```python
from build123d import *

# Parameters (mm, degrees)
F1_DEPTH = 20
F2_R     = 1.5
F3_DEPTH = 5.2010001


with BuildPart() as f1:
    # F0 (on Top) → F1 (new body)
    with BuildSketch(Plane.XY):
        with BuildLine():
            Line((-17.7, 10.1), (-17.7, 0))
            Line((-17.7, 0), (-17.7, -6.1))
            ThreePointArc((-17.7, -6.1), (-17.4363961031, -6.7363961031), (-16.8, -7))
            ThreePointArc((-16.8, -7), (-16.1636038969, -6.7363961031), (-15.9, -6.1))
            Line((-15.9, -6.1), (-15.9, -2.9281131564))
            Line((-15.9, -2.9281131564), (-15.9, -0.2))
            ThreePointArc((-15.9, -0.2), (-15.8414213562, -0.0585786438), (-15.7, 0))
            Line((-15.7, 0), (-13.1, 0))
            ThreePointArc((-13.1, 0), (-12.9585786438, -0.0585786438), (-12.9, -0.2))
            Line((-12.9, -0.2), (-12.9, -2.9281131564))
            Line((-12.9, -2.9281131564), (-12.9, -6.1))
            ThreePointArc((-12.9, -6.1), (-12.6363961031, -6.7363961031), (-12, -7))
            ThreePointArc((-12, -7), (-11.3636038969, -6.7363961031), (-11.1, -6.1))
            Line((-11.1, -6.1), (-11.1, -2.9281131564))
            ThreePointArc((-11.1, -2.9281131564), (-11.0414213562, -2.7866918002), (-10.9, -2.7281131564))
            Line((-10.9, -2.7281131564), (-10.7902640884, -2.7281131564))
            ThreePointArc((-10.7902640884, -2.7281131564), (-10.6130008648, -2.6207292974), (-10.6260897314, -2.4138906521))
            ThreePointArc((-10.6260897314, -2.4138906521), (-9.6, -0.45), (-8.5739102686, -2.4138906521))
            ThreePointArc((-8.5739102686, -2.4138906521), (-8.5869991352, -2.6207292974), (-8.4097359116, -2.7281131564))
            Line((-8.4097359116, -2.7281131564), (-8.3, -2.7281131564))
            ThreePointArc((-8.3, -2.7281131564), (-8.1585786438, -2.7866918002), (-8.1, -2.9281131564))
            Line((-8.1, -2.9281131564), (-8.1, -6.1))
            ThreePointArc((-8.1, -6.1), (-7.8363961031, -6.7363961031), (-7.2, -7))
            ThreePointArc((-7.2, -7), (-6.5636038969, -6.7363961031), (-6.3, -6.1))
            Line((-6.3, -6.1), (-6.3, -0.2))
            ThreePointArc((-6.3, -0.2), (-6.2414213562, -0.0585786438), (-6.1, 0))
            Line((-6.1, 0), (6.1, 0))
            ThreePointArc((6.1, 0), (6.2414213562, -0.0585786438), (6.3, -0.2))
            Line((6.3, -0.2), (6.3, -6.1))
            ThreePointArc((6.3, -6.1), (6.5636038969, -6.7363961031), (7.2, -7))
            ThreePointArc((7.2, -7), (7.8363961031, -6.7363961031), (8.1, -6.1))
            Line((8.1, -6.1), (8.1, -2.9281131564))
            ThreePointArc((8.1, -2.9281131564), (8.1585786438, -2.7866918002), (8.3, -2.7281131564))
            Line((8.3, -2.7281131564), (8.4097359116, -2.7281131564))
            ThreePointArc((8.4097359116, -2.7281131564), (8.5869991352, -2.6207292974), (8.5739102686, -2.4138906521))
            ThreePointArc((8.5739102686, -2.4138906521), (9.6, -0.45), (10.6260897314, -2.4138906521))
            ThreePointArc((10.6260897314, -2.4138906521), (10.6130008648, -2.6207292974), (10.7902640884, -2.7281131564))
            Line((10.7902640884, -2.7281131564), (10.9, -2.7281131564))
            ThreePointArc((10.9, -2.7281131564), (11.0414213562, -2.7866918002), (11.1, -2.9281131564))
            Line((11.1, -2.9281131564), (11.1, -6.1))
            ThreePointArc((11.1, -6.1), (11.3636038969, -6.7363961031), (12, -7))
            ThreePointArc((12, -7), (12.6363961031, -6.7363961031), (12.9, -6.1))
            Line((12.9, -6.1), (12.9, -2.9281131564))
            Line((12.9, -2.9281131564), (12.9, -0.2))
            ThreePointArc((12.9, -0.2), (12.9585786438, -0.0585786438), (13.1, 0))
            Line((13.1, 0), (15.7, 0))
            ThreePointArc((15.7, 0), (15.8414213562, -0.0585786438), (15.9, -0.2))
            Line((15.9, -0.2), (15.9, -2.9281131564))
            Line((15.9, -2.9281131564), (15.9, -6.1))
            ThreePointArc((15.9, -6.1), (16.1636038969, -6.7363961031), (16.8, -7))
            ThreePointArc((16.8, -7), (17.4363961031, -6.7363961031), (17.7, -6.1))
            Line((17.7, -6.1), (17.7, 0))
            Line((17.7, 0), (17.7, 10.1))
            ThreePointArc((17.7, 10.1), (17.4363961031, 10.7363961031), (16.8, 11))
            ThreePointArc((16.8, 11), (16.1636038969, 10.7363961031), (15.9, 10.1))
            Line((15.9, 10.1), (15.9, 2.2532098395))
            ThreePointArc((15.9, 2.2532098395), (15.8239660819, 2.096262681), (15.6536758945, 2.0586485965))
            Line((15.6536758945, 2.0586485965), (13.0536758945, 2.6776962156))
            ThreePointArc((13.0536758945, 2.6776962156), (12.9430528415, 2.7482913767), (12.9, 2.8722574585))
            Line((12.9, 2.8722574585), (12.9, 10.1))
            ThreePointArc((12.9, 10.1), (12.6363961031, 10.7363961031), (12, 11))
            ThreePointArc((12, 11), (11.3636038969, 10.7363961031), (11.1, 10.1))
            Line((11.1, 10.1), (11.1, 3.3960669823))
            ThreePointArc((11.1, 3.3960669823), (11.0239660819, 3.2391198239), (10.8536758945, 3.2015057394))
            Line((10.8536758945, 3.2015057394), (8.2536758945, 3.8205533584))
            ThreePointArc((8.2536758945, 3.8205533584), (8.1430528415, 3.8911485195), (8.1, 4.0151146014))
            Line((8.1, 4.0151146014), (8.1, 10.1))
            ThreePointArc((8.1, 10.1), (7.8363961031, 10.7363961031), (7.2, 11))
            ThreePointArc((7.2, 11), (6.5636038969, 10.7363961031), (6.3, 10.1))
            Line((6.3, 10.1), (6.3, 4.5389241252))
            ThreePointArc((6.3, 4.5389241252), (6.2239660819, 4.3819769667), (6.0536758945, 4.3443628823))
            Line((6.0536758945, 4.3443628823), (3.4536758945, 4.9634105013))
            ThreePointArc((3.4536758945, 4.9634105013), (3.3430528415, 5.0340056624), (3.3, 5.1579717442))
            Line((3.3, 5.1579717442), (3.3, 10.1))
            ThreePointArc((3.3, 10.1), (3.0363961031, 10.7363961031), (2.4, 11))
            ThreePointArc((2.4, 11), (1.7636038969, 10.7363961031), (1.5, 10.1))
            Line((1.5, 10.1), (1.5, 5.2))
            ThreePointArc((1.5, 5.2), (1.4414213562, 5.0585786438), (1.3, 5))
            Line((1.3, 5), (-1.3, 5))
            ThreePointArc((-1.3, 5), (-1.4414213562, 5.0585786438), (-1.5, 5.2))
            Line((-1.5, 5.2), (-1.5, 10.1))
            ThreePointArc((-1.5, 10.1), (-1.7636038969, 10.7363961031), (-2.4, 11))
            ThreePointArc((-2.4, 11), (-3.0363961031, 10.7363961031), (-3.3, 10.1))
            Line((-3.3, 10.1), (-3.3, 5.1579717442))
            ThreePointArc((-3.3, 5.1579717442), (-3.3430528415, 5.0340056624), (-3.4536758945, 4.9634105013))
            Line((-3.4536758945, 4.9634105013), (-6.0536758945, 4.3443628823))
            ThreePointArc((-6.0536758945, 4.3443628823), (-6.2239660819, 4.3819769667), (-6.3, 4.5389241252))
            Line((-6.3, 4.5389241252), (-6.3, 10.1))
            ThreePointArc((-6.3, 10.1), (-6.5636038969, 10.7363961031), (-7.2, 11))
            ThreePointArc((-7.2, 11), (-7.8363961031, 10.7363961031), (-8.1, 10.1))
            Line((-8.1, 10.1), (-8.1, 4.0151146014))
            ThreePointArc((-8.1, 4.0151146014), (-8.1430528415, 3.8911485195), (-8.2536758945, 3.8205533584))
            Line((-8.2536758945, 3.8205533584), (-10.8536758945, 3.2015057394))
            ThreePointArc((-10.8536758945, 3.2015057394), (-11.0239660819, 3.2391198239), (-11.1, 3.3960669823))
            Line((-11.1, 3.3960669823), (-11.1, 10.1))
            ThreePointArc((-11.1, 10.1), (-11.3636038969, 10.7363961031), (-12, 11))
            ThreePointArc((-12, 11), (-12.6363961031, 10.7363961031), (-12.9, 10.1))
            Line((-12.9, 10.1), (-12.9, 2.8722574585))
            ThreePointArc((-12.9, 2.8722574585), (-12.9430528415, 2.7482913767), (-13.0536758945, 2.6776962156))
            Line((-13.0536758945, 2.6776962156), (-15.6536758945, 2.0586485965))
            ThreePointArc((-15.6536758945, 2.0586485965), (-15.8239660819, 2.096262681), (-15.9, 2.2532098395))
            Line((-15.9, 2.2532098395), (-15.9, 10.1))
            ThreePointArc((-15.9, 10.1), (-16.1636038969, 10.7363961031), (-16.8, 11))
            ThreePointArc((-16.8, 11), (-17.4363961031, 10.7363961031), (-17.7, 10.1))
        make_face()
    extrude(amount=F1_DEPTH)

    # F2 (on face) → F3 (cut, through all)
    with BuildSketch(Plane.XZ):
        with Locations((0, 17)):
            Circle(F2_R)
    extrude(amount=-F3_DEPTH, mode=Mode.SUBTRACT)


solid = f1.part
```
Here's how the part is built. I have some questions about the finished solid (model axes, mm). A direction names the side the tool comes from. Give positions to 0.01 mm unless a question says otherwise; leave off trailing zeros. Order: outer loops, then holes, each group sorted by start corner. A loop starts at its lowest first (then second) coordinate and runs counter-clockwise, first axis right, second up. Notation, with made-up numbers: (-26, -34) - (33, -34) arc R17 cw to (33, -25) - close; hole circle Ø8 at (35, 10.5). An arc over 180 degrees is marked (long way). Answer as a JSON object with one key per item and string values. Group by question number.
Item 1: For P1, Ø2, axis at x = -9.6, y = -1.7, coming from the +Z side; P2, Ø3, axis at x = 0.5, z = 10.5, coming from the +Y side; P3, Ø3.5, axis at x = 0.5, z = 5.5, coming from the -Y side; P4, Ø1, axis at x = 11, z = 7, coming from the +Y side, each with a flat end and sliding along its axis, tell me the tip position at first contact or that it passes through.
Item 2: If we section it at D-D on x = -9.6: Please give me the cut outline in (y, z), and give its area (3 significant figures).
Item 3: If we section it at C-C on x = 0: Please give me the cut outline in (y, z), and give its area (3 significant figures).
Item 4: Which directions (+Z, -Z, +X, -X, +Y, -Y) give clear straight access to the entire face, cutting with the end or side of a thin tool? Please do faces 1 (the flat face through (-6.3, -3, 10)), 2 (the cylindrical face through (-9.64, -0.45, 9.86)), 3 (the flat face through (11.1, 7, 10)).
Item 5: If we section it at B-B on y = 9.5: Give the number of separate pieces and of enclosed holes in the cut face, and give its area (3 significant figures).
Item 6: If we mould it in two halves opening along X, with no side actions, what happens to faces 4 (the flat face through (1.5, 8, 10)), 5 (the flat face through (0, 2, 0)), 6 (the flat face through (11.1, -4, 10))? For each: pulls with the +X half, pulls with the -X half, needs draft (parallel to the pull), parting line crosses it, or undercut.
Item 7: Please list where these lines run through material, in increasing order: probe 1 along X at (y, z) = (-1.7, 12.5); probe 2 along X at (y, z) = (2.9, 17); probe 3 along X at (y, z) = (-2.5, 15.75).
Item 8: If we section it at A-A on y = -1.7: Please give me the cut outline in (x, z).
Result set:
{
 "1": {"P1": "through", "P2": "y = 10.91", "P3": "y = 0", "P4": "y = 10.85"},
 "2": {"outline": "(-0.45, 0) - (3.5, 0) - (3.5, 20) - (-0.45, 20) - close", "area": "79.0 mm²"},
 "3": {"outline": "(0, 0) - (5, 0) - (5, 15.5) - (0, 15.5) - close; (0, 18.5) - (5, 18.5) - (5, 20) - (0, 20) - close", "area": "85.0 mm²"},
 "4": {"face 1": "+Z, -Z, -Y", "face 2": "+Z, -Z", "face 3": "+Z, -Z, +Y"},
 "5": {"separate pieces": "8", "enclosed holes": "0", "area": "288 mm²"},
 "6": {"face 4": "undercut", "face 5": "needs draft", "face 6": "undercut"},
 "7": {"probe 1": "-17.7 to -15.9, -12.9 to -10.85, -8.35 to -6.3, 6.3 to 8.35, 10.85 to 12.9, 15.9 to 17.7", "probe 2": "-17.7 to -15.9, -12.9 to -1.5, 1.5 to 12.9, 15.9 to 17.7", "probe 3": "-17.7 to -15.9, -12.9 to -10.59, -8.61 to -6.3, 6.3 to 8.61, 10.59 to 12.9, 15.9 to 17.7"},
 "8": {"outline": "(-17.7, 0) - (-15.9, 0) - (-15.9, 20) - (-17.7, 20) - close; (-12.9, 0) - (-10.85, 0) - (-10.85, 20) - (-12.9, 20) - close; (-8.35, 0) - (-6.3, 0) - (-6.3, 20) - (-8.35, 20) - close; (6.3, 0) - (8.35, 0) - (8.35, 20) - (6.3, 20) - close; (10.85, 0) - (12.9, 0) - (12.9, 20) - (10.85, 20) - close; (15.9, 0) - (17.7, 0) - (17.7, 20) - (15.9, 20) - close"}
}
